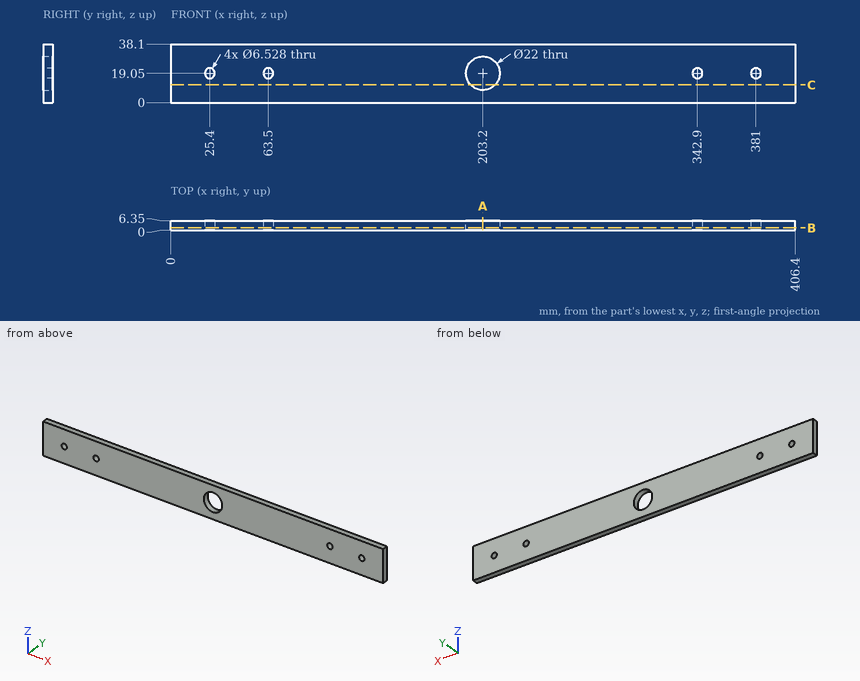
Verification items for this drawing (mm, ordinates from the low corner). Coordinates: 2 decimals unless noted, no trailing zeros. Write each loop counter-clockwise with the first axis right and the second up, starting at its lowest first coordinate (ties: lowest second). Pieces come first, ordered by that corner, then holes. Notation, with made-up numbers: M -17,72.5 L -6,72.5 A36 cw -6,109.5 Z; hole C 49.5,-25 d10. An arc over 180 degrees is marked long. Answer as CSV lines item,"result".
Q1. Material ranges on probe 1 along X at (y, z) = (3.75, 17.5); probe 2 along X at (y, z) = (3.5, 12); probe 3 along X at (y, z) = (1.5, 14), recorded low to high. Write a range as from..to.
Check result:
probe 1,"0..22.53, 28.27..60.63, 66.37..192.31, 214.09..340.03, 345.77..378.13, 383.87..406.4"
probe 2,"0..194.76, 211.64..406.4"
probe 3,"0..193.43, 212.97..406.4"
Q2. Cross-section at B-B (y = 1.5). Record the boundary of the cut face in (x, z), then the cut area to 3 significant figures.
Check result:
outline,"M 0,0 L 406.4,0 L 406.4,38.1 L 0,38.1 Z; hole C 25.4,19.05 d6.53; hole C 63.5,19.05 d6.53; hole C 203.2,19.05 d22; hole C 342.9,19.05 d6.53; hole C 381,19.05 d6.53"
area,"15,000 mm^2"
Q3. Cross-section at A-A (x = 203.2). Record the boundary of the cut face in (y, z).
Check result:
outline,"M 0,0 L 6.35,0 L 6.35,8.05 L 0,8.05 Z; M 0,30.05 L 6.35,30.05 L 6.35,38.1 L 0,38.1 Z"
Q4. Go/stop test with a flat-tipped pin: pin 1 (17.5 mm diameter, centred on x = 203.2, z = 19.05, fed in from -Y). Record where the tip stops, or that it passes through.
Check result:
pin 1,"through"
Q5. Cross-section at C-C (z = 11.5). Record the boundary of the cut face in (x, y), then the cut area to 3 significant figures.
Check result:
outline,"M 0,0 L 195.2,0 L 195.2,6.35 L 0,6.35 Z; M 211.2,0 L 406.4,0 L 406.4,6.35 L 211.2,6.35 Z"
area,"2,480 mm^2"
